Could you check a few things on this model? Use its own coordinates, in mm. Face numbers are marked on the shaded views. A direction names the side the tool comes from. Give positions to 0.01 mm unless a question says otherwise; leave off trailing zeros. Loops run counter-clockwise (first coordinate to the right, second up) from the corner with the lowest first, then second, coordinate; pieces in that order, holes last. Notation, with made-up numbers: (16.5, -12) - (63.5, -12) arc R8 ccw to (63.5, -6) - close; hole circle Ø1 at (44, 0). An arc over 180 degrees is marked (long way). Answer in a Markdown table with one row per item. Add a question column.
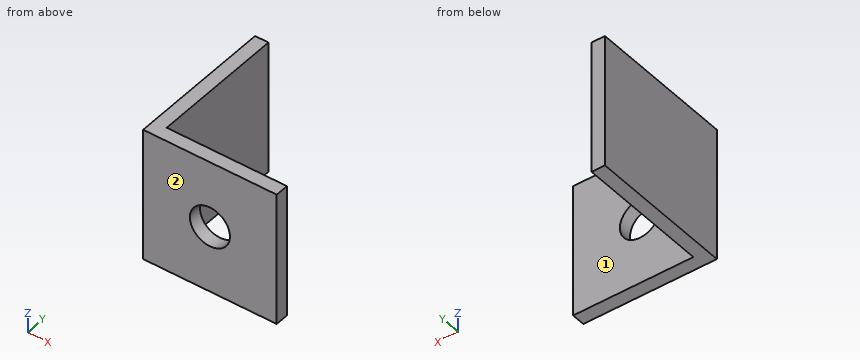
```python
from build123d import *

# Parameters (mm, degrees)
SKETCH_2_W      = 20
SKETCH_2_H      = 20
SKETCH_2_R      = 3
EXTRUDE_1_DEPTH = 2
SKETCH_3_W      = 2
SKETCH_3_H      = 20
EXTRUDE_2_DEPTH = 20


with BuildPart() as part:
    # ｽｹｯﾁ2 → ﾎﾞｽ - 押し出し1 (new body)
    with BuildSketch(Plane(origin=(0, 0, 0), x_dir=(1, 0, 0), z_dir=(0, 1, 0))):
        Rectangle(SKETCH_2_W, SKETCH_2_H)
        with Locations(Location((0, 0, 0), (0, 0, 270))):
            Circle(SKETCH_2_R, mode=Mode.SUBTRACT)
    extrude(amount=EXTRUDE_1_DEPTH)

    # ｽｹｯﾁ3 → ﾎﾞｽ - 押し出し2 (add)
    with BuildSketch(Plane(origin=(0, 2, 0), x_dir=(1, 0, 0), z_dir=(0, 1, 0))):
        with Locations((-9, 0)):
            Rectangle(SKETCH_3_W, SKETCH_3_H)
    extrude(amount=EXTRUDE_2_DEPTH)


solid = part.part
```
(1) I want a section at B-B on x = 2.25. Please give me the cut outline in (y, z), then the cut area to 3 significant figures.
(2) I want a section at D-D on z = 4.5. Please give me the cut outline in (x, y), then the cut area to 3 significant figures.
(3) Please list where these lines run through material, in increasing order: line 1 (X direction, y = 0.6, z = 0); line 2 (Y direction, x = 0.75, z = -5.5); line 3 (X direction, y = 8.5, z = -2.75).
(4) I want a section at C-C on y = 1.5. Please give me the cut outline in (x, z), then the cut area to 3 significant figures.
(5) For pin 1 Ø7 at (x, z) = (0, 0) entering from +Y; pin 2 Ø5 at (y, z) = (15, -2.5) entering from +X, each with a flat end and sliding along its axis, tell me the tip position at first contact or that it passes through.
(6) I want a section at A-A on z = 0. Please give me the cut outline in (x, y).
(7) On a 3-axis mill with a long thin cutter (end or side, diameter ignored), from which of +Z, -Z, +X, -X, +Y, -Y can I reach the whole of each face in a straight line? I mean the marked faces 1 and 2. Say none if no direction works.
Reported:
| question | item | result |
|---|---|---|
| 1 | outline | (0, -10) - (2, -10) - (2, -1.98) - (0, -1.98) - close; (0, 1.98) - (2, 1.98) - (2, 10) - (0, 10) - close |
| 1 | area | 32.1 mm² |
| 2 | outline | (-10, 0) - (10, 0) - (10, 2) - (-8, 2) - (-8, 22) - (-10, 22) - close |
| 2 | area | 80.0 mm² |
| 3 | line 1 | -10 to -3, 3 to 10 |
| 3 | line 2 | 0 to 2 |
| 3 | line 3 | -10 to -8 |
| 4 | outline | (-10, -10) - (10, -10) - (10, 10) - (-10, 10) - close; hole circle Ø6 at (0, 0) |
| 4 | area | 372 mm² |
| 5 | pin 1 | y = 2 |
| 5 | pin 2 | x = -8 |
| 6 | outline | (-10, 0) - (-3, 0) - (-3, 2) - (-8, 2) - (-8, 22) - (-10, 22) - close; (3, 0) - (10, 0) - (10, 2) - (3, 2) - close |
| 7 | face 1 | +Z, -Z, +X, +Y |
| 7 | face 2 | +Z, -Z, +X, -X, -Y |
